Model file for the job. Use its own axes, mm. Face numbers are marked on the shaded views. Coordinates: 2 decimals unless noted, no trailing zeros. Write each loop counter-clockwise with the first axis right and the second up, starting at its lowest first coordinate (ties: lowest second). Pieces come first, ordered by that corner, then holes. Notation, with made-up numbers: (64.5, 16.25) -> (90.5, 16.25) arc R24 ccw to (90.5, 42.25) -> close; hole circle Ø5 at (20.25, -17.5). An arc over 180 degrees is marked (long way). Write item = value, one per line. Start each with the question number.
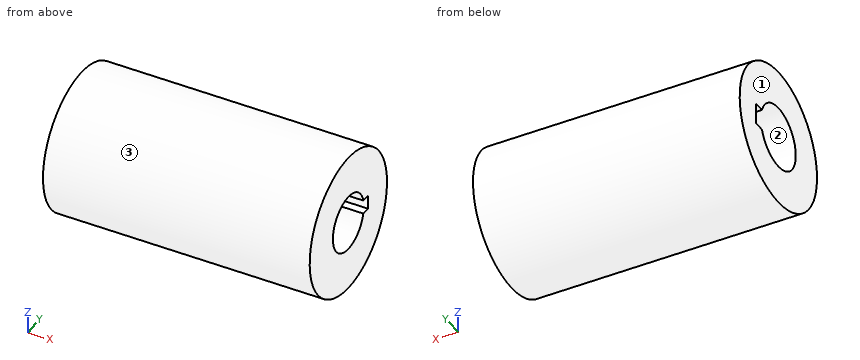
from build123d import *

# Parameters (mm, degrees)
SKETCH1_R           = 10
BOSS_EXTRUDE2_DEPTH = 38
SKETCH9_R           = 4
CUT_EXTRUDE5_DEPTH  = 38
SKETCH10_R          = 4.5
CUT_EXTRUDE6_DEPTH  = 18
SKETCH11_W          = 3
SKETCH11_H          = 1.6
CUT_EXTRUDE7_DEPTH  = 18
SKETCH12_W          = 2
SKETCH12_H          = 1.2
CUT_EXTRUDE8_DEPTH  = 20


with BuildPart() as part:
    # Sketch1 → Boss-Extrude2 (new body)
    with BuildSketch(Plane(origin=(0, 0, 0), x_dir=(0, 0, -1), z_dir=(1, 0, 0))):
        Circle(SKETCH1_R)
    extrude(amount=BOSS_EXTRUDE2_DEPTH)

    # Sketch9 → Cut-Extrude5 (cut)
    with BuildSketch(Plane(origin=(38, 0, 0), x_dir=(0, 0, -1), z_dir=(1, 0, 0))):
        Circle(SKETCH9_R)
    extrude(amount=-CUT_EXTRUDE5_DEPTH, mode=Mode.SUBTRACT)

    # Sketch10 → Cut-Extrude6 (cut)
    with BuildSketch(Plane.ZY):
        Circle(SKETCH10_R)
    extrude(amount=-CUT_EXTRUDE6_DEPTH, mode=Mode.SUBTRACT)

    # Sketch11 → Cut-Extrude7 (cut)
    with BuildSketch(Plane.ZY):
        with Locations((0, 5.042640687)):
            Rectangle(SKETCH11_W, SKETCH11_H)
    extrude(amount=-CUT_EXTRUDE7_DEPTH, mode=Mode.SUBTRACT)

    # Sketch12 → Cut-Extrude8 (cut)
    with BuildSketch(Plane(origin=(38, 0, 0), x_dir=(0, 0, -1), z_dir=(1, 0, 0))):
        with Locations((0, 4.472983346)):
            Rectangle(SKETCH12_W, SKETCH12_H)
    extrude(amount=-CUT_EXTRUDE8_DEPTH, mode=Mode.SUBTRACT)


solid = part.part
(1) Mould opens along Y. For the marked faces 1, 2 and 3 say: released by +Y, released by -Y, zero draft, split by the parting line, or undercut.
(2) Drill centre lines: line 1 along Y through (x, z) = (19, 0); line 2 along Y through (x, z) = (4.75, 0); line 3 along Z through (x, y) = (11, 3.25). Where is each one in solid material? Low to high.
(3) Saw through at B-B (z = 0). Give the cut face in (x, y).
(4) Saw through at C-C (x = 30.5). Give the cut face in (y, z), then the cut area to 3 significant figures.
(5) Saw through at D-D (y = 8). Give the cut face in (x, z), then the cut area to 3 significant figures.
(6) Saw through at A-A (y = 0). Give the cut face in (x, z), then the cut area to 3 significant figures.
(7) Drop flat-ended pins along their axis: pin 1 Ø10 at (x, z) = (6.5, 6.5) entering from -Y; pin 2 Ø4.5 at (y, z) = (-1, 0) entering from -X; pin 3 Ø3 at (x, z) = (18, 4) entering from -Y; pin 4 Ø1 at (x, y) = (25, 4.5) entering from +Z. Give the stop position or say it passes through.
Returned:
q1.face_1 = zero draft
q1.face_2 = undercut
q1.face_3 = split by the parting line
q2.line_1 = -10 to -4, 5.07 to 10
q2.line_2 = -10 to -4.5, 5.84 to 10
q2.line_3 = -9.46 to -3.11, 3.11 to 9.46
q3.outline = (0, -10) -> (38, -10) -> (38, -4) -> (18, -4) -> (18, -4.5) -> (0, -4.5) -> close; (0, 5.84) -> (18, 5.84) -> (18, 5.07) -> (38, 5.07) -> (38, 10) -> (0, 10) -> close
q4.outline = circle Ø20 at (0, 0); hole (3.87, -1) -> (5.07, -1) -> (5.07, 1) -> (3.87, 1) arc R4 ccw (long way) to start
q4.area = 262 mm2
q5.outline = (0, -6) -> (38, -6) -> (38, 6) -> (0, 6) -> close
q5.area = 456 mm2
q6.outline = (0, -10) -> (38, -10) -> (38, -4) -> (18, -4) -> (18, -4.5) -> (0, -4.5) -> close; (0, 4.5) -> (18, 4.5) -> (18, 4) -> (38, 4) -> (38, 10) -> (0, 10) -> close
q6.area = 438 mm2
q7.pin_1 = -9.89
q7.pin_2 = through
q7.pin_3 = -9.68
q7.pin_4 = 9.17
